Input: part model. Units: mm. Frame: model coordinates. A direction names the side the tool comes from. Coordinates: 2 decimals unless noted, no trailing zeros. Loops run counter-clockwise (first coordinate to the right, second up) from the corner with the lowest first, then second, coordinate; pieces in that order, holes last. Notation, with made-up numbers: (53, -28.75) - (85, -28.75) arc R35 cw to (85, 8.25) - close; hole circle Ø1 at (20.25, 81). An arc over 180 degrees is marked (long way). Write item = value, one per line. Start each with the question number.
from build123d import *

# Parameters (mm, degrees)
SKETCH_1_R      = 12.5
SKETCH_1_R_2    = 6
EXTRUDE_1_DEPTH = 9.5
EXTRUDE_2_DEPTH = 10


with BuildPart() as part:
    # 草图1 → 凸台-拉伸1 (new body)
    with BuildSketch(Plane.XY):
        Circle(SKETCH_1_R)
        Circle(SKETCH_1_R_2, mode=Mode.SUBTRACT)
    extrude(amount=EXTRUDE_1_DEPTH)

    # 草图2 → 凸台-拉伸2 (add)
    with BuildSketch(Plane(origin=(0, 0, 0), x_dir=(-1, 0, 0), z_dir=(0, 0, -1))):
        with BuildLine():
            Line((7.846282243, -1.560722576), (12.259816005, -2.438629025))
            ThreePointArc((12.259816005, -2.438629025), (12.5, 0), (12.259816005, 2.438629025))
            Line((12.259816005, 2.438629025), (7.846282243, 1.560722576))
            ThreePointArc((7.846282243, 1.560722576), (8, 0), (7.846282243, -1.560722576))
        make_face()
        with BuildLine():
            Line((1.560722576, 7.846282243), (2.438629025, 12.259816005))
            ThreePointArc((2.438629025, 12.259816005), (0, 12.5), (-2.438629025, 12.259816005))
            Line((-2.438629025, 12.259816005), (-1.560722576, 7.846282243))
            ThreePointArc((-1.560722576, 7.846282243), (0, 8), (1.560722576, 7.846282243))
        make_face()
        with BuildLine():
            Line((-1.560722576, -7.846282243), (-2.438629025, -12.259816005))
            ThreePointArc((-2.438629025, -12.259816005), (0, -12.5), (2.438629025, -12.259816005))
            Line((2.438629025, -12.259816005), (1.560722576, -7.846282243))
            ThreePointArc((1.560722576, -7.846282243), (0, -8), (-1.560722576, -7.846282243))
        make_face()
        with BuildLine():
            Line((-7.846282243, 1.560722576), (-12.259816005, 2.438629025))
            ThreePointArc((-12.259816005, 2.438629025), (-12.5, 0), (-12.259816005, -2.438629025))
            Line((-12.259816005, -2.438629025), (-7.846282243, -1.560722576))
            ThreePointArc((-7.846282243, -1.560722576), (-8, 0), (-7.846282243, 1.560722576))
        make_face()
    extrude(amount=EXTRUDE_2_DEPTH)


solid = part.part
Item 1: Pin query (flat end, axial travel): pin 1 (4 mm diameter, centred on y = -4, z = 5, fed in from -X); pin 2 (6 mm diameter, centred on x = -6.5, z = -1.5, fed in from -Y); pin 3 (2 mm diameter, centred on y = -3.5, z = 2.5, fed in from +X). Return the tip coordinate at first contact, or that it passes through.
Item 2: Access query for faces 4 (the flat face through (-2.006, -10.084, -4.93)), 5 (the flat face through (10.022, 1.994, -4.93)), 6 (the flat face through (-10.022, -1.994, -4.93)), 7 (the flat face through (2.006, 10.084, -4.93)), 8 (the cylindrical face through (0, 8, -5)). Directions: +Z, -Z, +X, -X, +Y, -Y. A direction counts if a zero-diameter tool reaches every point of the face in a straight line with its end or side. Return the directions, or none.
Item 3: Ray query, line 1 (Y direction, x = 0, z = 4.75); line 2 (X direction, y = 1.5, z = 8.75); line 3 (X direction, y = -1.5, z = -5). Return the intervals inside material, ascending.
Item 4: Pull-direction query (Y, two-part tool) for faces 1 (the flat face through (-3, -5.4, 9.5)), 2 (the flat face through (-10.084, 2.006, -4.93)), 3 (the flat face through (-1.994, 10.022, -4.93)); classes: pulls with the +Y half, pulls with the -Y half, needs draft (parallel to the pull), parting line crosses it, or undercut.
Item 5: Cut plane B-B on y = 0. Return loops of the section in (x, z).
Item 6: Cut plane A-A on z = -6.25. Return loops of the section in (x, y), plus the area to 3 significant figures.
Item 7: Cut plane D-D on x = 11. Return loops of the section in (y, z), plus the area to 3 significant figures.
Recorded:
q1.pin_1 = -12.34
q1.pin_2 = -11.88
q1.pin_3 = 12.25
q2.face_4 = -Z, -X
q2.face_5 = -Z, +Y
q2.face_6 = -Z, -Y
q2.face_7 = -Z, +X
q2.face_8 = -Z
q3.line_1 = -12.5 to -6, 6 to 12.5
q3.line_2 = -12.41 to -5.81, 5.81 to 12.41
q3.line_3 = -12.41 to -7.86, 7.86 to 12.41
q4.face_1 = needs draft
q4.face_2 = pulls with the +Y half
q4.face_3 = undercut
q5.outline = (-12.5, -10) - (-8, -10) - (-8, 0) - (-6, 0) - (-6, 9.5) - (-12.5, 9.5) - close; (6, 0) - (8, 0) - (8, -10) - (12.5, -10) - (12.5, 9.5) - (6, 9.5) - close
q6.outline = (-12.26, -2.44) - (-7.85, -1.56) arc R8 cw to (-7.85, 1.56) - (-12.26, 2.44) arc R12.5 ccw to start; (-2.44, -12.26) arc R12.5 ccw to (2.44, -12.26) - (1.56, -7.85) arc R8 cw to (-1.56, -7.85) - close; (-2.44, 12.26) - (-1.56, 7.85) arc R8 cw to (1.56, 7.85) - (2.44, 12.26) arc R12.5 ccw to start; (7.85, -1.56) - (12.26, -2.44) arc R12.5 ccw to (12.26, 2.44) - (7.85, 1.56) arc R8 cw to start
q6.area = 72.5 mm²
q7.outline = (-5.94, 0) - (-2.19, 0) - (-2.19, -10) - (2.19, -10) - (2.19, 0) - (5.94, 0) - (5.94, 9.5) - (-5.94, 9.5) - close
q7.area = 157 mm²
